Model file for the job. Use its own axes, mm. A direction names the side the tool comes from. Coordinates: 2 decimals unless noted, no trailing zeros. Order: outer loops, then holes, each group sorted by start corner. A loop starts at its lowest first (then second) coordinate and runs counter-clockwise, first axis right, second up. Notation, with made-up numbers: (21.5, 46.5) -> (30.5, 46.5) arc R6 ccw to (30.5, 53.5) -> close; hole circle Ø9 at (-21.5, -14). An arc over 180 degrees is marked (long way). Return JSON: item names as keys, results as strings. Group by question number.
1) Cut at D-D (x = -26.67). Write the cut outline in (y, z) (3 decimals), and give its area (3 significant figures).
2) Flat gauge pins, fed straight in: pin 1 (10 mm diameter, centred on x = -39, z = 47, fed in from -Y); pin 2 (2 mm diameter, centred on x = 55, z = -65.5, fed in from +Y). Where does each tip first touch, or does it go through?
3) Pull direction Z, two halves, no side cores. Call faces 4 (the flat face through (-1, 0, -2)), 5 (the flat face through (-1, 5, -114.3)), 6 (the cylindrical face through (45.26, 5.8, 102.75)): +Z half, -Z half, draft (parallel to the pull), parting line (faces both ways), or undercut.
4) Which spindle directions (+Z, -Z, +X, -X, +Y, -Y) get a long thin tool onto all of the face, cutting with end or side? Do faces 1 (the flat face through (-88.9, 5, 2)), 2 (the cylindrical face through (-45.79, 5.587, 5.725)), 3 (the cylindrical face through (8.96, 5.587, 35.423)). Say none if no direction does.
5) Cut at B-B (x = 63.5). Write the cut outline in (y, z) (3 decimals), and give its area (3 significant figures).
6) Cut at C-C (z = -92.71). Write the cut outline in (x, y) (3 decimals), and give its area (3 significant figures).
7) Probe line 1 (Z direction, x = 46.5, y = 8.25); line 2 (Z direction, x = 41, y = 9) (3 decimals); line 3 (Z direction, x = 52.5, y = 6.75). List the from-to ranges inside material, lowest first.
from build123d import *

# Parameters (mm, degrees)
SKETCH1_W           = 177.8
SKETCH1_H           = 228.6
BOSS_EXTRUDE1_DEPTH = 10.16


with BuildPart() as part:
    # Sketch1 → Boss-Extrude1 (new body)
    with BuildSketch(Plane(origin=(0, 0, 0), x_dir=(1, 0, 0), z_dir=(0, 1, 0))):
        Rectangle(SKETCH1_W, SKETCH1_H)
    extrude(amount=BOSS_EXTRUDE1_DEPTH)

    # Cut-Sweep2: sweep along a path in Sketch2
    with BuildLine(Plane(origin=(0, 10.16, 0), x_dir=(1, 0, 0), z_dir=(0, 1, 0))) as cut_sweep2_path:
        Line((8.89, -114.3), (8.89, 38.1))
        Line((8.89, 38.1), (0, 38.1))
        Line((0, 38.1), (0, -92.71))
        Line((0, -92.71), (-8.89, -92.71))
        Line((-8.89, -92.71), (-8.89, 46.99))
        Line((-8.89, 46.99), (17.78, 46.99))
        Line((17.78, 46.99), (17.78, -101.6))
        Line((17.78, -101.6), (26.67, -101.6))
        Line((26.67, -101.6), (26.67, 55.88))
        Line((26.67, 55.88), (-17.78, 55.88))
        Line((-17.78, 55.88), (-17.78, -92.71))
        Line((-17.78, -92.71), (-26.67, -92.71))
        Line((-26.67, -92.71), (-26.67, 64.77))
        Line((-26.67, 64.77), (35.56, 64.77))
        Line((35.56, 64.77), (35.56, -101.6))
        Line((35.56, -101.6), (54.61, -101.6))
        Line((54.61, -101.6), (54.61, 83.82))
        Line((54.61, 83.82), (-45.72, 83.82))
        Line((-45.72, 83.82), (-45.72, -92.71))
        Line((-45.72, -92.71), (-54.61, -92.71))
        Line((-54.61, -92.71), (-54.61, 92.71))
        Line((-54.61, 92.71), (63.5, 92.71))
        Line((63.5, 92.71), (63.5, -101.6))
        Line((63.5, -101.6), (72.39, -101.6))
        Line((72.39, -101.6), (72.39, 101.6))
        Line((72.39, 101.6), (-63.5, 101.6))
        Line((-63.5, 101.6), (-63.5, -101.6))
        Line((-63.5, -101.6), (-8.89, -101.6))
        Line((-8.89, -101.6), (-8.89, -114.3))
    # Sketch4 → Cut-Sweep2 (sweep, cut)
    with BuildSketch(Plane.XY.offset(114.3)):
        with BuildLine():
            Line((-5.715, 10.16), (-5.715, 8.760933946))
            ThreePointArc((-5.715, 8.760933946), (-8.89, 5.585933946), (-12.065, 8.760933946))
            Line((-12.065, 8.760933946), (-12.065, 10.16))
            ThreePointArc((-12.065, 10.16), (-8.89, 13.335), (-5.715, 10.16))
        make_face()
    sweep(path=cut_sweep2_path.line, transition=Transition.RIGHT, mode=Mode.SUBTRACT)


solid = part.part
Answers below:
{
 "1": {"outline": "(0, -114.3) -> (10.16, -114.3) -> (10.16, -104.775) -> (8.761, -104.775) arc R3.175 cw to (8.761, -98.425) -> (10.16, -98.425) -> (10.16, -95.885) -> (8.761, -95.885) arc R3.175 cw to (8.761, -89.535) -> (10.16, -89.535) -> (10.16, -86.995) -> (8.761, -86.995) arc R3.175 cw to (8.761, -80.645) -> (10.16, -80.645) -> (10.16, -67.945) -> (8.761, -67.945) arc R3.175 cw to (5.586, -64.77) -> (5.586, 92.71) arc R3.175 cw to (8.761, 95.885) -> (10.16, 95.885) -> (10.16, 98.425) -> (8.761, 98.425) arc R3.175 cw to (8.761, 104.775) -> (10.16, 104.775) -> (10.16, 114.3) -> (0, 114.3) -> close", "area": "1,480 mm^2"},
 "2": {"pin 1": "stops at y = 0", "pin 2": "stops at y = 5.91"},
 "3": {"face 4": "draft", "face 5": "-Z half", "face 6": "undercut"},
 "4": {"face 1": "+Z, -Z, -X, +Y, -Y", "face 2": "+Y", "face 3": "+Z, +Y"},
 "5": {"outline": "(0, -114.3) -> (10.16, -114.3) -> (10.16, -104.775) -> (8.761, -104.775) arc R3.175 cw to (8.761, -98.425) -> (10.16, -98.425) -> (10.16, -95.885) -> (8.761, -95.885) arc R3.175 cw to (5.586, -92.71) -> (5.586, 101.6) arc R3.175 cw to (8.761, 104.775) -> (10.16, 104.775) -> (10.16, 114.3) -> (0, 114.3) -> close", "area": "1,380 mm^2"},
 "6": {"outline": "(-88.9, 0) -> (88.9, 0) -> (88.9, 10.16) -> (75.565, 10.16) -> (75.565, 8.761) arc R3.175 cw to (69.215, 8.761) -> (69.215, 10.16) -> (66.675, 10.16) -> (66.675, 8.761) arc R3.175 cw to (63.5, 5.586) -> (-54.61, 5.586) arc R3.175 cw to (-57.785, 8.761) -> (-57.785, 10.16) -> (-60.325, 10.16) -> (-60.325, 8.761) arc R3.175 cw to (-66.675, 8.761) -> (-66.675, 10.16) -> (-88.9, 10.16) -> close", "area": "1,190 mm^2"},
 "7": {"line 1": "z = -114.3 to -104.73, -98.47 to -95.84, -89.58 to -86.95, -80.69 to 98.47, 104.73 to 114.3", "line 2": "z = -114.3 to -104.775, -98.425 to -95.885, -89.535 to -86.995, -80.645 to 98.425, 104.775 to 114.3", "line 3": "z = -114.3 to -104.06, -99.14 to -95.17, -90.25 to -86.28, 104.06 to 114.3"}
}
